Input: part model. Units: mm. Frame: model coordinates. Face numbers are marked on the shaded views. Coordinates: 2 decimals unless noted, no trailing zeros. Loops run counter-clockwise (first coordinate to the right, second up) from the corner with the lowest first, then second, coordinate; pieces in that order, holes last.
Item 1: Ray query, line 1 along Y through (x, z) = (0, 3.7); line 2 along X through (y, z) = (-10.5, 1.5); line 3 along X through (y, z) = (-8, 0.25). Return the intervals inside material, ascending.
Item 2: Pull-direction query (X, two-part tool) for the marked faces 1 and 2; classes: released by +X, released by -X, zero draft, split by the parting line, or undercut.
Item 3: Section B-B on x = -8. Return loops of the section in (y, z), and give its area (3 significant figures).
Item 4: Section A-A on x = -34. Return loops of the section in (y, z).
Item 5: Section D-D on x = 13.5. Return loops of the section in (y, z), and give its area (3 significant figures).
Item 6: Section C-C on x = 23. Return loops of the section in (y, z), and give its area (3 significant figures).
Item 7: Contact query for flat-ended pins moving along their axis: P1, Ø2, axis at x = 0, y = 0, coming from the +Z side; P2, Ø3, axis at x = 17, y = 29.44, coming from the +Z side; P3, Ø4, axis at x = 19.5, z = 2.5, coming from the -Y side; P4, Ø1, axis at x = 25.5, z = -1, coming from the -Y side. Output: stop coordinate, or through.
```python
from build123d import *

# Parameters (mm, degrees)
SKETCH_1_R                       = 32.1
EXTRUDE_1_DEPTH                  = 5
EXTRUDE_START                    = 0.8
SKETCH_2_R                       = 36.5
EXTRUDE_2_DEPTH                  = 1.6
SKETCH_3_R                       = 38.5
EXTRUDE_3_DEPTH                  = 2
SKETCH_4_R                       = 26.1
CUT_EXTRUDE_1_DEPTH              = 56.003090822
SKETCH_4_3_R                     = 5
EXTRUDE_4_DEPTH                  = 7.8
EXTRUDE_5_DEPTH                  = 7.8
FILLET_6_R                       = 2
PATTERN_CIRCULAR_2_COUNT         = 6
FILLET_6_OF_PATTERN_CIRCULAR_2_R = 2
FILLET_7_R                       = 10
SKETCH_6_R                       = 0.75
CUT_EXTRUDE_2_DEPTH              = 3
SKETCH_8_R                       = 1
CUT_EXTRUDE_4_DEPTH              = 55.608973622
SKETCH_8_3_R                     = 1.75
CUT_EXTRUDE_5_DEPTH              = 2.1


with BuildPart() as part:
    # Sketch 1 → Extrude 1 (new body)
    with BuildSketch(Plane.XY):
        Circle(SKETCH_1_R)
    extrude(amount=EXTRUDE_1_DEPTH)

    # Sketch 2 → Extrude 2 (add)
    with BuildSketch(Plane(origin=(0, 0, 0), x_dir=(-1, 0, 0), z_dir=(0, 0, -1)).offset(EXTRUDE_START)):
        Circle(SKETCH_2_R)
    extrude(amount=-EXTRUDE_2_DEPTH)

    # Sketch 3 → Extrude 3 (add)
    with BuildSketch(Plane(origin=(0, 0, -0.8), x_dir=(-1, 0, 0), z_dir=(0, 0, -1))):
        Circle(SKETCH_3_R)
    extrude(amount=EXTRUDE_3_DEPTH)

    # Sketch 4 → Cut-Extrude 1 (cut, through all)
    with BuildSketch(Plane.XY.offset(5)):
        Circle(SKETCH_4_R)
    extrude(amount=-CUT_EXTRUDE_1_DEPTH, mode=Mode.SUBTRACT)



with BuildPart() as body_2:
    # Sketch 4_3 → Extrude 4 (new, through all)
    with BuildSketch(Plane.XY.offset(5)):
        Circle(SKETCH_4_3_R)
    extrude(amount=-EXTRUDE_4_DEPTH)


with BuildPart() as part_1:
    add(part.part)

    add(body_2.part)  # Extrude 5 merges body 2
    # Sketch 4_4 → Extrude 5 (add, through all)
    with BuildSketch(Plane.XY.offset(5)):
        with BuildLine():
            Line((-1.820643965, 26.036421712), (-0.348782369, 4.987820251))
            ThreePointArc((-0.348782369, 4.987820251), (0, 5), (0.348782369, 4.987820251))
            Line((0.348782369, 4.987820251), (1.820643965, 26.036421712))
            ThreePointArc((1.820643965, 26.036421712), (0, 26.1), (-1.820643965, 26.036421712))
        make_face()
    extrude_5 = extrude(amount=-EXTRUDE_5_DEPTH)

    # Fillet 6
    fillet_6_edges = [part_1.edges().sort_by_distance(p)[0] for p in [
        (1.820643965, 26.036421712, 1.1),
        (-1.820643965, 26.036421712, 1.1),
    ]]
    fillet(fillet_6_edges, radius=FILLET_6_R)

    # Pattern Circular 2: Extrude 5 ×6 about axis
    pattern_circular_2_axis = Axis((0, 0, 0), (0, 0, 1))
    for i in range(1, PATTERN_CIRCULAR_2_COUNT):
        add(extrude_5.rotate(pattern_circular_2_axis, i * 360 / PATTERN_CIRCULAR_2_COUNT))

    # Fillet 6 of Pattern Circular 2
    fillet_6_of_pattern_circular_2_edges = [part_1.edges().sort_by_distance(p)[0] for p in [
        (-21.637880644, 14.594934781, 1.1),
        (-23.458524608, 11.441486931, 1.1),
        (-23.458524608, -11.441486931, 1.1),
        (-21.637880644, -14.594934781, 1.1),
        (-1.820643965, -26.036421712, 1.1),
        (1.820643965, -26.036421712, 1.1),
        (21.637880644, -14.594934781, 1.1),
        (23.458524608, -11.441486931, 1.1),
        (23.458524608, 11.441486931, 1.1),
        (21.637880644, 14.594934781, 1.1),
    ]]
    fillet(fillet_6_of_pattern_circular_2_edges, radius=FILLET_6_OF_PATTERN_CIRCULAR_2_R)

    # Fillet 7
    # the kernel refuses this fillet: 10 mm, written as the material it adds along each edge
    with BuildSketch(Plane(origin=(-4.493970231, -2.191855734, 5), x_dir=(-0.8987940462991628, -0.4383711467890857, 0), z_dir=(0, 0, -1)), Plane(origin=(-0.348782369, -4.987820251, 5), x_dir=(-0.06975647374411581, -0.9975640502598249, 0), z_dir=(0, 0, -1)), Plane(origin=(4.145187863, -2.795964517, 5), x_dir=(0.8290375725550467, -0.5591929034707394, 0), z_dir=(0, 0, -1)), Plane(origin=(4.493970231, 2.191855734, 5), x_dir=(0.8987940462991627, 0.43837114678908606, 0), z_dir=(0, 0, -1)), Plane(origin=(0.348782369, 4.987820251, 5), x_dir=(0.0697564737441158, 0.9975640502598249, 0), z_dir=(0, 0, -1)), Plane(origin=(-4.145187863, 2.795964517, 5), x_dir=(-0.8290375725550471, 0.5591929034707388, 0), z_dir=(0, 0, -1))) as fillet_7_piece_1:
        with BuildLine():
            CenterArc((6.180339887, 10), FILLET_7_R, 221.810314896, 48.189685104)
            ThreePointArc((-1.273220038, 3.333333333), (-0.329138205, 1.784110449), (0, 0))
            Line((0, 0), (6.180339887, 0))
        make_face()
    extrude(amount=7.8)
    with BuildSketch(Plane(origin=(-4.145187863, -2.795964517, 5), x_dir=(-0.8290375725550488, -0.5591929034707364, 0), z_dir=(0, 0, -1)), Plane(origin=(0.348782369, -4.987820251, 5), x_dir=(0.06975647374411298, -0.9975640502598251, 0), z_dir=(0, 0, -1)), Plane(origin=(4.493970231, -2.191855734, 5), x_dir=(0.8987940462991613, -0.4383711467890891, 0), z_dir=(0, 0, -1)), Plane(origin=(4.145187863, 2.795964517, 5), x_dir=(0.8290375725550484, 0.5591929034707368, 0), z_dir=(0, 0, -1)), Plane(origin=(-0.348782369, 4.987820251, 5), x_dir=(-0.0697564737441132, 0.9975640502598251, 0), z_dir=(0, 0, -1)), Plane(origin=(-4.493970231, 2.191855734, 5), x_dir=(-0.8987940462991615, 0.43837114678908873, 0), z_dir=(0, 0, -1))) as fillet_7_piece_2:
        with BuildLine():
            CenterArc((6.180339887, -10), FILLET_7_R, 90, 48.189685104)
            ThreePointArc((-1.273220038, -3.333333333), (-0.329138205, -1.784110449), (0, 0))
            Line((0, 0), (6.180339887, 0))
        make_face()
    extrude(amount=7.8)

    # Sketch 6 → Cut-Extrude 2 (cut)
    with BuildSketch(Plane.XY.offset(5)):
        Circle(SKETCH_6_R)
        with Locations((-14.55, 25.20133925)):
            Circle(SKETCH_6_R)
        with Locations((29.1, 0)):
            Circle(SKETCH_6_R)
        with Locations((-14.55, -25.20133925)):
            Circle(SKETCH_6_R)
    extrude(amount=-CUT_EXTRUDE_2_DEPTH, mode=Mode.SUBTRACT)

    # Sketch 8 → Cut-Extrude 4 (cut, through all)
    with BuildSketch(Plane.XY.offset(0.8)):
        with Locations((17, 29.444863729)):
            Circle(SKETCH_8_R)
        with Locations((-34, 0)):
            Circle(SKETCH_8_R)
        with Locations((17, -29.444863729)):
            Circle(SKETCH_8_R)
    extrude(amount=-CUT_EXTRUDE_4_DEPTH, mode=Mode.SUBTRACT)

    # Sketch 8_3 → Cut-Extrude 5 (cut)
    with BuildSketch(Plane.XY.offset(0.8)):
        with Locations((-34, 0)):
            Circle(SKETCH_8_3_R)
        with Locations((17, 29.444863729)):
            Circle(SKETCH_8_3_R)
        with Locations((17, -29.444863729)):
            Circle(SKETCH_8_3_R)
    extrude(amount=-CUT_EXTRUDE_5_DEPTH, mode=Mode.SUBTRACT)


solid = part_1.part
```
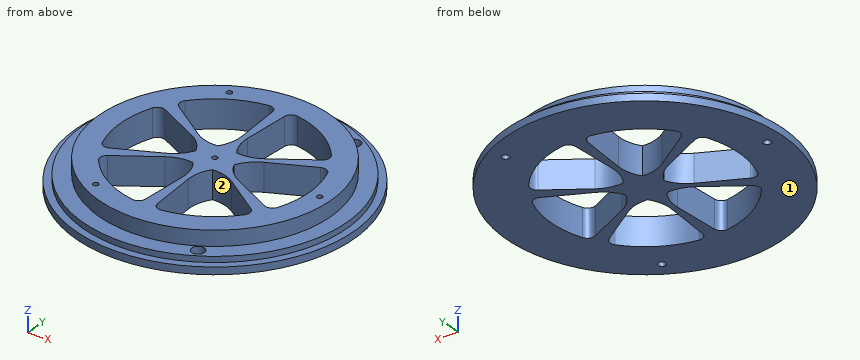
Results found:
1. line 1: y = -32.1 to -0.75, 0.75 to 32.1
1. line 2: x = -30.33 to -23.4, -21.53 to -15.57, -0.76 to 0.76, 15.57 to 21.53, 23.4 to 30.33
1. line 3: x = -35.61 to -24.84, -16.4 to -11.86, -1.06 to 1.06, 11.86 to 16.4, 24.84 to 35.61
2. face 1: zero draft
2. face 2: undercut
3. outline: (-37.66, -2.8) - (-24.84, -2.8) - (-24.84, 5) - (-31.09, 5) - (-31.09, 0.8) - (-35.61, 0.8) - (-35.61, -0.8) - (-37.66, -0.8) - close; (-5.53, -2.8) - (-3.57, -2.8) - (-3.57, 5) - (-5.53, 5) - close; (3.57, -2.8) - (5.53, -2.8) - (5.53, 5) - (3.57, 5) - close; (24.84, -2.8) - (37.66, -2.8) - (37.66, -0.8) - (35.61, -0.8) - (35.61, 0.8) - (31.09, 0.8) - (31.09, 5) - (24.84, 5) - close
3. area: 169 mm2
4. outline: (-18.06, -2.8) - (-1, -2.8) - (-1, -1.3) - (-1.75, -1.3) - (-1.75, 0.8) - (-13.28, 0.8) - (-13.28, -0.8) - (-18.06, -0.8) - close; (1, -2.8) - (18.06, -2.8) - (18.06, -0.8) - (13.28, -0.8) - (13.28, 0.8) - (1.75, 0.8) - (1.75, -1.3) - (1, -1.3) - close
5. outline: (-36.06, -2.8) - (-22.34, -2.8) - (-22.34, 5) - (-29.12, 5) - (-29.12, 0.8) - (-33.91, 0.8) - (-33.91, -0.8) - (-36.06, -0.8) - close; (-9.11, -2.8) - (-6.58, -2.8) - (-6.58, 5) - (-9.11, 5) - close; (6.58, -2.8) - (9.11, -2.8) - (9.11, 5) - (6.58, 5) - close; (22.34, -2.8) - (36.06, -2.8) - (36.06, -0.8) - (33.91, -0.8) - (33.91, 0.8) - (29.12, 0.8) - (29.12, 5) - (22.34, 5) - close
5. area: 188 mm2
6. outline: (-30.87, -2.8) - (-10.66, -2.8) - (-10.66, 5) - (-22.39, 5) - (-22.39, 0.8) - (-28.34, 0.8) - (-28.34, -0.8) - (-30.87, -0.8) - close; (10.66, -2.8) - (30.87, -2.8) - (30.87, -0.8) - (28.34, -0.8) - (28.34, 0.8) - (22.39, 0.8) - (22.39, 5) - (10.66, 5) - close
6. area: 236 mm2
7. P1: stops at z = 5
7. P2: stops at z = -1.3
7. P3: stops at y = -31.5
7. P4: stops at y = -29.28
